Check sheet for the modelled part. Datum: model origin and axes. Units: mm. Give positions to 0.01 mm unless a question says otherwise; leave off trailing zeros. Order: outer loops, then holes, each group sorted by start corner. A loop starts at its lowest first (then second) coordinate and runs counter-clockwise, first axis right, second up.
Item 1: Material ranges on line 1 along Y through (x, z) = (-5, 3.3); line 2 along Y through (x, z) = (4, 3.95); line 3 along Y through (x, z) = (-13, 0.7), recorded low to high.
Item 2: Gauge pin test, flat ends, axial feed: P1, Ø5.5, axis at x = -5, y = -8.43, coming from the +Z side; P2, Ø2, axis at x = -5, y = -187.57, coming from the -Z side. Record the tip position at first contact, or that the pin passes through.
Item 3: Sectioned sample at B-B on z = 1.3. Record the boundary of the cut face in (x, y), and give its area (3 significant figures).
Item 4: Sectioned sample at A-A on x = -5. Record the boundary of the cut face in (y, z).
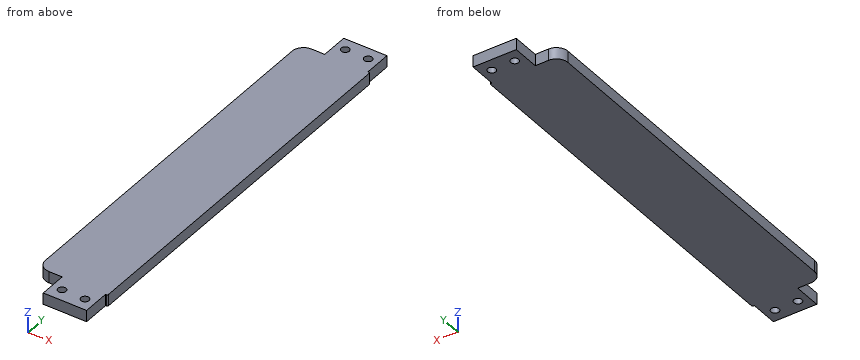
from build123d import *

# Parameters (mm, degrees)
SKETCH1_R           = 1.75
BOSS_EXTRUDE1_DEPTH = 5


with BuildPart() as part:
    # Sketch1 → Boss-Extrude1 (new body)
    with BuildSketch(Plane.XY):
        with BuildLine():
            Line((-20.194136312, -20), (-20.194136312, -176))
            ThreePointArc((-20.194136312, -176), (-18.729670218, -179.535533906), (-15.194136312, -181))
            Line((-15.194136312, -181), (-9.446581599, -181))
            Line((-9.446581599, -181), (-9.446581599, -193))
            Line((-9.446581599, -193), (9.446581599, -193))
            Line((9.446581599, -193), (9.446581599, -181))
            Line((9.446581599, -181), (9.846581599, -181))
            ThreePointArc((9.846581599, -181), (10.200134989, -180.853553391), (10.346581599, -180.5))
            Line((10.346581599, -180.5), (10.346581599, -15.5))
            ThreePointArc((10.346581599, -15.5), (10.200134989, -15.146446609), (9.846581599, -15))
            Line((9.846581599, -15), (9.446581599, -15))
            Line((9.446581599, -15), (9.446581599, -3))
            Line((9.446581599, -3), (-9.413759597, -3))
            Line((-9.413759597, -3), (-9.413759597, -15))
            Line((-9.413759597, -15), (-15.194136312, -15))
            ThreePointArc((-15.194136312, -15), (-18.729670218, -16.464466094), (-20.194136312, -20))
        make_face()
        with Locations((-5, -187.570297721)):
            Circle(SKETCH1_R, mode=Mode.SUBTRACT)
        with Locations((5, -187.570297721)):
            Circle(SKETCH1_R, mode=Mode.SUBTRACT)
        with Locations((-5, -8.429702279)):
            Circle(SKETCH1_R, mode=Mode.SUBTRACT)
        with Locations((5, -8.429702279)):
            Circle(SKETCH1_R, mode=Mode.SUBTRACT)
    extrude(amount=BOSS_EXTRUDE1_DEPTH)


solid = part.part
Report:
1. line 1: y = -193 to -189.32, -185.82 to -10.18, -6.68 to -3
1. line 2: y = -193 to -189.01, -186.13 to -9.87, -6.99 to -3
1. line 3: y = -181 to -15
2. P1: stops at z = 5
2. P2: passes through
3. outline: (-20.19, -176) arc R5 ccw to (-15.19, -181) - (-9.45, -181) - (-9.45, -193) - (9.45, -193) - (9.45, -181) - (9.85, -181) arc R0.5 ccw to (10.35, -180.5) - (10.35, -15.5) arc R0.5 ccw to (9.85, -15) - (9.45, -15) - (9.45, -3) - (-9.41, -3) - (-9.41, -15) - (-15.19, -15) arc R5 ccw to (-20.19, -20) - close; hole circle Ø3.5 at (-5, -187.57); hole circle Ø3.5 at (-5, -8.43); hole circle Ø3.5 at (5, -187.57); hole circle Ø3.5 at (5, -8.43)
3. area: 5,470 mm2
4. outline: (-193, 0) - (-189.32, 0) - (-189.32, 5) - (-193, 5) - close; (-185.82, 0) - (-10.18, 0) - (-10.18, 5) - (-185.82, 5) - close; (-6.68, 0) - (-3, 0) - (-3, 5) - (-6.68, 5) - close
